```python
from build123d import *

# Parameters (mm, degrees)
SKETCH_1_R          = 6
EXTRUDE_1_DEPTH     = 6
CUT_EXTRUDE_1_DEPTH = 10


with BuildPart() as part:
    # 草图1 → 凸台-拉伸1 (new body)
    with BuildSketch(Plane(origin=(0, 0, 0), x_dir=(0, 0, -1), z_dir=(1, 0, 0))):
        with BuildLine():
            Line((15, 0), (17.5, -200))
            ThreePointArc((17.5, -200), (0, -217.5), (-17.5, -200))
            Line((-17.5, -200), (-15, 0))
            ThreePointArc((-15, 0), (0, 15), (15, 0))
        make_face()
        Circle(SKETCH_1_R, mode=Mode.SUBTRACT)
        with Locations((0, -200)):
            Circle(SKETCH_1_R, mode=Mode.SUBTRACT)
    extrude(amount=EXTRUDE_1_DEPTH)

    # 草图2 → 切除-拉伸1 (cut)
    with BuildSketch(Plane(origin=(6, 0, 0), x_dir=(0, 0, -1), z_dir=(1, 0, 0))):
        with BuildLine():
            Line((5, -25), (5, -85))
            ThreePointArc((5, -85), (0, -90), (-5, -85))
            Line((-5, -85), (-5, -25))
            ThreePointArc((-5, -25), (0, -20), (5, -25))
        make_face()
        with BuildLine():
            Line((4.5, -105), (4.5, -160))
            ThreePointArc((4.5, -160), (0, -164.5), (-4.5, -160))
            Line((-4.5, -160), (-4.5, -105))
            ThreePointArc((-4.5, -105), (0, -100.5), (4.5, -105))
        make_face()
    extrude(amount=-CUT_EXTRUDE_1_DEPTH, mode=Mode.SUBTRACT)


solid = part.part
```
Part model, mm, in its own coordinate system. A direction names the side the tool comes from. Give positions to 0.01 mm unless a question says otherwise; leave off trailing zeros. Order: outer loops, then holes, each group sorted by start corner. A loop starts at its lowest first (then second) coordinate and runs counter-clockwise, first axis right, second up. Notation, with made-up numbers: M 33,20 L 92,20 A3 cw 92,24 Z; hole C -28,-39.5 d8. An arc over 180 degrees is marked long. Use a Markdown table: item, result. Add a question column.
(1) 3-axis set-ups, long thin cutter, end or side, ignore diameter. For faces 1 (the face through (3, -20, 0)), 2 (the face through (0, -100, 0)): which of +Z, -Z, +X, -X, +Y, -Y reach the whole face in a straight line?
(2) Probe line 1 along Y through (x, z) = (2.1, 0); line 2 along Z through (x, y) = (1.15, -49.5); line 3 along Z through (x, y) = (1.8, -30) (3 decimals). List the from-to ranges inside material, lowest first. Write a range as [from, to].
(3) Saw through at D-D, the plane y = -2.5. Give the cut face in (x, z), and give its area (3 significant figures).
(4) Drop flat-ended pins along their axis: P1, Ø1.8, axis at x = 4, y = -146, coming from the -Z side; P2, Ø3, axis at x = 3, y = -123, coming from the +Z side; P3, Ø9.5, axis at y = -200, z = 0, coming from the +X side; P4, Ø15.5, axis at y = 0, z = 0, coming from the +X side. Give the stop position or say it passes through.
(5) Saw through at B-B, the plane z = 0. Give the cut face in (x, y).
(6) Mould opens along Y. For faces 3 (the face through (3, 15, 0)), 4 (the face through (3, -100.5, 0.1)), 5 (the face through (6, -100, 0)) say: +Y half, -Y half, draft (parallel to the pull), parting line (faces both ways), or undercut.
(7) Saw through at C-C, the plane x = 3.2. Give the cut face in (y, z), and give its area (3 significant figures).
(8) Saw through at A-A, the plane y = -144. Give the cut face in (x, z).
Answer key:
| question | item | result |
|---|---|---|
| 1 | face 1 | +X, -X |
| 1 | face 2 | +Z, -Z, -X, +Y, -Y |
| 2 | line 1 | [-217.5, -206], [-194, -164.5], [-100.5, -90], [-20, -6], [6, 15] |
| 2 | line 2 | [-15.62, -5], [5, 15.62] |
| 2 | line 3 | [-15.375, -5], [5, 15.375] |
| 3 | outline | M 0,-15.03 L 6,-15.03 L 6,-5.45 L 0,-5.45 Z; M 0,5.45 L 6,5.45 L 6,15.03 L 0,15.03 Z |
| 3 | area | 115 mm^2 |
| 4 | P1 | z = -16.84 |
| 4 | P2 | z = 16.56 |
| 4 | P3 | through |
| 4 | P4 | x = 6 |
| 5 | outline | M 0,-217.5 L 6,-217.5 L 6,-206 L 0,-206 Z; M 0,-194 L 6,-194 L 6,-164.5 L 0,-164.5 Z; M 0,-100.5 L 6,-100.5 L 6,-90 L 0,-90 Z; M 0,-20 L 6,-20 L 6,-6 L 0,-6 Z; M 0,6 L 6,6 L 6,15 L 0,15 Z |
| 6 | face 3 | +Y half |
| 6 | face 4 | undercut |
| 6 | face 5 | draft |
| 7 | outline | M -200,-17.5 L 0,-15 A15 ccw 0,15 L -200,17.5 A17.5 ccw Z; hole C -200,0 d12; hole M -160,-4.5 L -105,-4.5 A4.5 ccw -105,4.5 L -160,4.5 A4.5 ccw Z; hole M -85,-5 L -25,-5 A5 ccw -25,5 L -85,5 A5 ccw Z; hole C 0,0 d12 |
| 7 | area | 5,870 mm^2 |
| 8 | outline | M 0,-16.8 L 6,-16.8 L 6,-4.5 L 0,-4.5 Z; M 0,4.5 L 6,4.5 L 6,16.8 L 0,16.8 Z |
